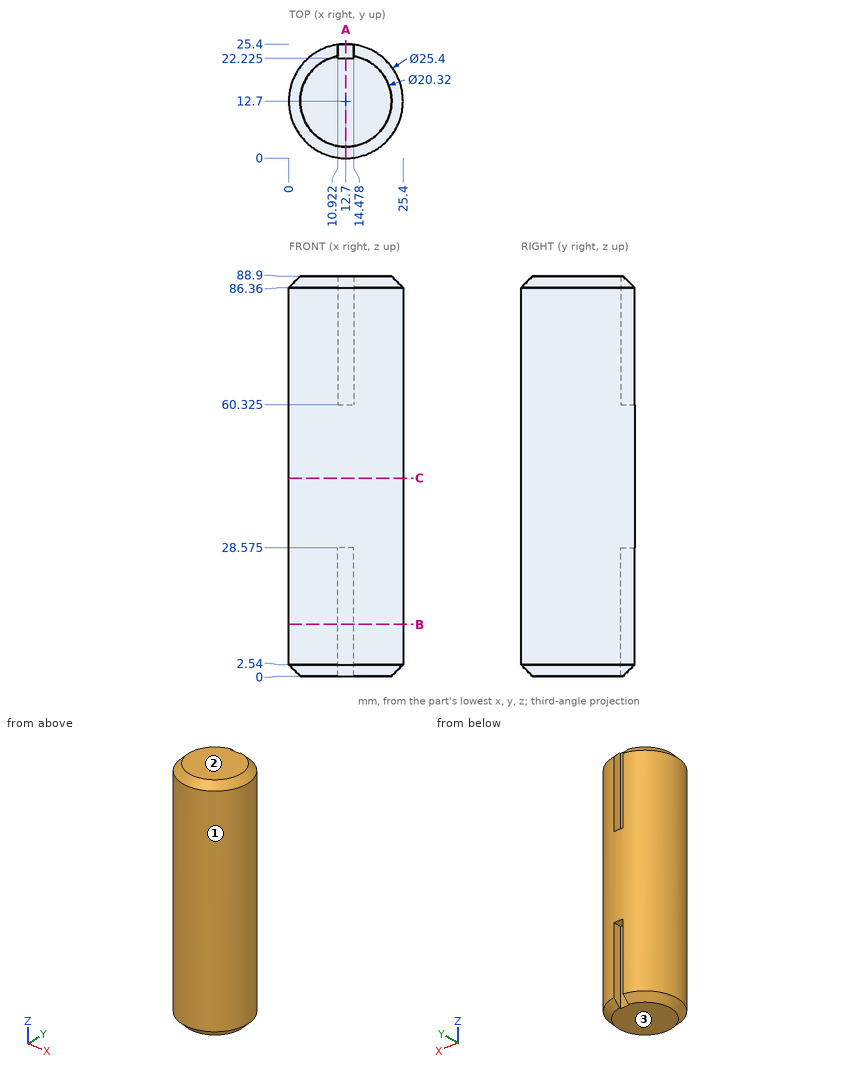
Print and shaded views of the part. All mm, measured from the part's lowest x, y and z. Coordinates: 2 decimals unless noted, no trailing zeros. Order: outer loops, then holes, each group sorted by start corner. A loop starts at its lowest first (then second) coordinate and runs counter-clockwise, first axis right, second up. Notation, with made-up numbers: M 21.25,79.25 L 64.25,79.25 A29 ccw 64.25,107.25 Z; hole C 26,78 d4. An arc over 180 degrees is marked long. Write each question's results on one line, items separated by ' | '. Start each with the question number.
Q1. Pull direction Z, two halves, no side cores. Call the marked faces 1, 2 and 3: +Z half, -Z half, draft (parallel to the pull), parting line (faces both ways), or undercut.
Q2. Flat gauge pins, fed straight in: P1, Ø12, axis at y = 4.5, z = 65, coming from the +X side; P2, Ø1, axis at x = 10, y = 16.5, coming from the -Z side; P3, Ø2.5, axis at y = 23.5, z = 19, coming from the +X side; P4, Ø2.5, axis at y = 24.5, z = 18.5, coming from the -X side. Where does each tip first touch, or does it go through?
Q3. Cut at A-A (x = 12.7). List the corners of the cut face in (y, z) (3 decimals).
Q4. Drill centre lines: probe 1 along Y at (x, z) = (12.5, 20) (3 decimals); probe 2 along Z at (x, y) = (11.75, 22.5) (3 decimals); probe 3 along Y at (x, z) = (15.25, 48.5). Where is each one in solid material? Low to high. Write a range as from..to.
Q5. Cut at B-B (z = 11.5). List the corners of the cut face in (x, y) (3 decimals).
Q6. Cut at C-C (z = 44). List the corners of the cut face in (x, y), then the cut area to 3 significant figures.
Found:
1) face 1: draft | face 2: +Z half | face 3: -Z half
2) P1: x = 25.21 | P2: z = 0 | P3: x = 21.07 | P4: x = 5.63
3) outline: M 0,2.54 L 2.54,0 L 22.225,0 L 22.225,28.575 L 25.4,28.575 L 25.4,60.325 L 22.225,60.325 L 22.225,88.9 L 2.54,88.9 L 0,86.36 Z
4) probe 1: 0.002..22.225 | probe 2: 28.575..60.325 | probe 3: 0.26..25.14
5) outline: M 10.922,22.225 L 10.922,25.275 A12.7 ccw long 14.478,25.275 L 14.478,22.225 Z
6) outline: C 12.7,12.7 d25.4 | area: 507 mm²
